Geometry: final body of the model. Coordinates: model frame, mm. Face numbers are marked on the shaded views. Round coordinates to 2 decimals unless told otherwise and drop trailing zeros. Write each loop counter-clockwise with the first axis right and the second up, starting at its lowest first coordinate (ties: lowest second). Pieces come first, ordered by that corner, then holes. Notation, with made-up numbers: (0.25, 4.25) -> (50.25, 4.25) arc R21 cw to (50.25, 19.25) -> close; hole circle Ø4 at (-22, 17.5). An arc over 180 degrees is marked (long way). One line per item, written item: value. Start each with the question number.
from build123d import *

# Parameters (mm, degrees)
SKETCH1_W           = 50
SKETCH1_H           = 40
BOSS_EXTRUDE1_DEPTH = 40
CUT_LOFT1_START     = -23.040884378
CUT_LOFT1_DEPTH     = 41.231056256


# Read off the part's stored shape, not the designer's step: Cut-Loft1
with BuildPart() as part:
    # Sketch1 → Boss-Extrude1 (new body)
    with BuildSketch(Plane(origin=(0, 0, 0), x_dir=(1, 0, 0), z_dir=(0, 1, 0))):
        Rectangle(SKETCH1_W, SKETCH1_H)
    extrude(amount=BOSS_EXTRUDE1_DEPTH)

    # Cut-Loft1 outline → Cut-Loft1 (cut)
    with BuildSketch(Plane(origin=(0, 0, 0), x_dir=(0.6859943405700354, 0.5144957554275265, -0.5144957554275265), z_dir=(0.7276068751089988, -0.4850712500726662, 0.4850712500726662)).offset(CUT_LOFT1_START)):
        Polygon((-1.908261965, 44), (0, 42.426406871), (17.149858514, 28.284271247), (42.874646286, 21.213203436), (44, 20.903873287), (44, 44), align=None)
    extrude(amount=CUT_LOFT1_DEPTH, mode=Mode.SUBTRACT)


solid = part.part
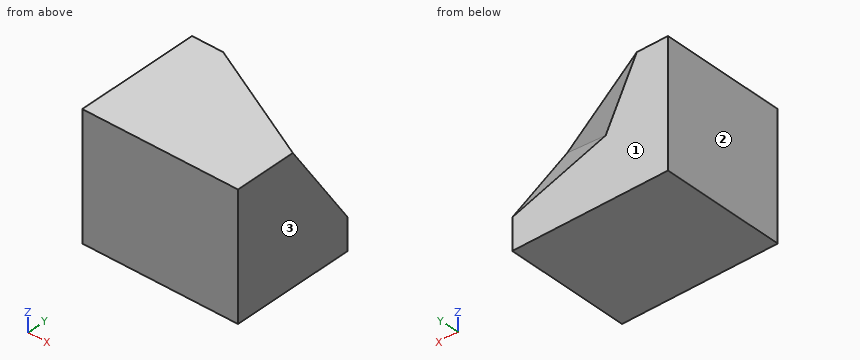
(1) Section query C-C (z = -4). Output: boundary loops of the cut face in (x, y).
(2) Section query B-B (x = 11.5). Output: boundary loops of the cut face in (y, z), and give its area (3 significant figures).
(3) Section query A-A (y = 36.5). Output: boundary loops of the cut face in (x, z).
(4) Section query D-D (x = -7). Output: boundary loops of the cut face in (y, z), and give its area (3 significant figures).
(5) Pull-direction query (X, two-part tool) for the marked faces 1, 2 and 3; classes: pulls with the +X half, pulls with the -X half, needs draft (parallel to the pull), parting line crosses it, or undercut.
(6) Line query: probe 1 along Y at (x, z) = (14, -0.5); probe 2 along Y at (x, z) = (9, 8); probe 3 along X at (y, z) = (37.5, 18.5). Output: solid intervals per line, ascending.
(7) Pin query (flat end, axial travel): pin 1 (5 mm diameter, centred on x = 13.5, z = 13, fed in from +Y). Return the tip coordinate at first contact, or that it passes through.
Results list:
1. outline: (-25, 0) -> (25, 0) -> (25, 36) -> (7, 40) -> (-25, 40) -> close
2. outline: (0, -20) -> (40, -20) -> (40, -5.5) -> (29, 11) -> (26.75, 20) -> (0, 20) -> close
2. area: 1,400 mm^2
3. outline: (-25, -20) -> (25, -20) -> (25, -4.75) -> (0.25, 3.5) -> (-8, 20) -> (-25, 20) -> close
4. outline: (0, -20) -> (40, -20) -> (40, 4) -> (36, 20) -> (0, 20) -> close
4. area: 1,570 mm^2
5. face 1: needs draft
5. face 2: pulls with the -X half
5. face 3: pulls with the +X half
6. probe 1: y = 0 to 36.11
6. probe 2: y = 0 to 31.56
6. probe 3: x = -25 to -9.25
7. pin 1: stops at y = 28.98
